Can you work these out from the model? Positions are in its coordinate system, mm. A direction names the side the tool comes from. Round coordinates to 2 decimals unless told otherwise and drop trailing zeros. Loops run counter-clockwise (first coordinate to the right, second up) from the corner with the lowest first, then second, coordinate; pieces in that order, holes last.
Autodesk Inventor part; units mm, degrees
ref_plane "YZ Plane" through (0, 0, 0) normal (1, 0, 0) x (0, 1, 0)
ref_plane "XZ Plane" through (0, 0, 0) normal (0, 1, 0) x (-1, 0, 0)
ref_plane "XY Plane" through (0, 0, 0) normal (0, 0, 1) x (1, 0, 0)
sketch "Sketch1" plane through (0, 0, 0) normal (0, 1, 0) x (-1, 0, 0)
  line L0 (-114.3, 114.3) -> (114.3, 114.3)
  line L1 (114.3, 114.3) -> (114.3, -114.3)
  line L2 (114.3, -114.3) -> (-114.3, -114.3)
  line L3 (-114.3, -114.3) -> (-114.3, 114.3)
  line L4 (-114.3, 114.3) -> (114.3, -114.3) construction
  line L5 (114.3, 114.3) -> (-114.3, -114.3) construction
  line L6 (114.3, 114.3) -> (38.1, 114.3)
  line L7 (38.1, 114.3) -> (38.1, 76.2) construction
  line L8 (38.1, 76.2) -> (114.3, 76.2) construction
  line L9 (114.3, 76.2) -> (114.3, 114.3)
  circle A0 centre (38.1, 76.2) radius 1.5875
  line L10 (114.3, 0) -> (47.3217, 0)
  line L11 (-114.3, 114.3) -> (-38.1, 114.3)
  line L12 (-38.1, 114.3) -> (-38.1, 76.2) construction
  line L13 (-38.1, 76.2) -> (-114.3, 76.2) construction
  line L14 (-114.3, 76.2) -> (-114.3, 114.3)
  circle A1 centre (-38.1, 76.2) radius 1.5875
  line L15 (-114.3, -114.3) -> (-38.1, -114.3)
  line L16 (-38.1, -114.3) -> (-38.1, -76.2) construction
  line L17 (-38.1, -76.2) -> (-114.3, -76.2) construction
  line L18 (-114.3, -76.2) -> (-114.3, -114.3)
  line L19 (114.3, -114.3) -> (38.1, -114.3)
  line L20 (38.1, -114.3) -> (38.1, -76.2) construction
  line L21 (38.1, -76.2) -> (114.3, -76.2) construction
  line L22 (114.3, -76.2) -> (114.3, -114.3)
  circle A2 centre (-38.1, -76.2) radius 1.5875
  circle A3 centre (38.1, -76.2) radius 1.5875
  point P0 (0, 0)
  dimension "d0" = 228.6
  dimension "d1" = 228.6
  dimension "d2" = 76.2
  dimension "d3" = 38.1
  dimension "d4" = 3.175
  dimension "d5" = 76.2
  dimension "d6" = 3.175
  dimension "d7" = 38.1
  dimension "d8" = 76.2
  dimension "d9" = 3.175
  dimension "d10" = 3.175
extrude "Extrusion1" add sketch "Sketch1" along normal blind 12.7
fillet "Fillet1" radius 3.175 4 edges at (-114.3, 6.35, 114.3) (114.3, 6.35, 114.3) (114.3, 6.35, -114.3) (-114.3, 6.35, -114.3)
sketch "Sketch4" plane through (0, 12.7, 0) normal (0, 1, 0) x (1, 0, 0)
  circle A0 centre (-38.1, 76.2) radius 1.5875
  circle A1 centre (38.1, 76.2) radius 1.5875
  circle A2 centre (38.1, -76.2) radius 1.5875
  circle A3 centre (-38.1, -76.2) radius 1.5875
  arc A4 (-111.125, 114.3) -> (-114.3, 111.125) centre (-111.125, 111.125) ccw
  line L0 (-114.3, 111.125) -> (-114.3, -111.125)
  arc A5 (-114.3, -111.125) -> (-111.125, -114.3) centre (-111.125, -111.125) ccw
  line L1 (-111.125, -114.3) -> (111.125, -114.3)
  arc A6 (111.125, -114.3) -> (114.3, -111.125) centre (111.125, -111.125) ccw
  line L2 (114.3, -111.125) -> (114.3, 111.125)
  arc A7 (114.3, 111.125) -> (111.125, 114.3) centre (111.125, 111.125) ccw
  line L3 (111.125, 114.3) -> (-111.125, 114.3)
  line L4 (114.3, 114.3) -> (73.025, 114.3) construction
  line L5 (73.025, 114.3) -> (73.025, 107.95) construction
  line L6 (73.025, 107.95) -> (114.3, 107.95) construction
  line L7 (114.3, 107.95) -> (114.3, 114.3) construction
  line L8 (114.3, 114.3) -> (73.025, 114.3) construction
  line L9 (73.025, 114.3) -> (73.025, 57.15) construction
  line L10 (73.025, 57.15) -> (114.3, 57.15) construction
  line L11 (114.3, 57.15) -> (114.3, 114.3) construction
  circle A8 centre (73.025, 57.15) radius 1.5875
  circle A9 centre (73.025, 107.95) radius 1.5875
  point P0 (0, 0)
  dimension "d22" = 41.275
  dimension "d23" = 6.35
  dimension "d24" = 57.15
  dimension "d25" = 3.175
  dimension "d26" = 3.175
extrude "camMount" cut sketch "Sketch4" against normal up to surface (12.7 mm away) contours A8 | A9
sketch "Sketch5" plane through (0, 12.7, 0) normal (0, 1, 0) x (1, 0, 0)
  circle A0 centre (73.025, 57.15) radius 1.5875 construction
  circle A1 centre (73.025, 107.95) radius 1.5875 construction
  circle A2 centre (-38.1, 76.2) radius 1.5875 construction
  circle A3 centre (38.1, 76.2) radius 1.5875 construction
  circle A4 centre (38.1, -76.2) radius 1.5875 construction
  circle A5 centre (-38.1, -76.2) radius 1.5875 construction
  arc A6 (-111.125, 114.3) -> (-114.3, 111.125) centre (-111.125, 111.125) ccw construction
  line L0 (-114.3, 111.125) -> (-114.3, -111.125) construction
  arc A7 (-114.3, -111.125) -> (-111.125, -114.3) centre (-111.125, -111.125) ccw construction
  line L1 (-111.125, -114.3) -> (111.125, -114.3) construction
  arc A8 (111.125, -114.3) -> (114.3, -111.125) centre (111.125, -111.125) ccw construction
  line L2 (114.3, -111.125) -> (114.3, 111.125) construction
  arc A9 (114.3, 111.125) -> (111.125, 114.3) centre (111.125, 111.125) ccw construction
  line L3 (111.125, 114.3) -> (-111.125, 114.3) construction
  line L4 (114.3, -114.3) -> (107.95, -114.3) construction
  line L5 (107.95, -77.089) -> (114.3, -77.089) construction
  line L6 (114.3, -77.089) -> (114.3, -114.3) construction
  line L7 (114.3, -114.3) -> (59.6392, -114.3) construction
  line L8 (59.6392, -77.089) -> (114.3, -77.089) construction
  line L9 (114.3, -77.089) -> (114.3, -114.3) construction
  line L10 (114.3, -114.3) -> (27.8892, -114.3) construction
  line L11 (27.8892, -114.3) -> (27.8892, -77.089) construction
  line L12 (27.8892, -77.089) -> (114.3, -77.089) construction
  line L13 (114.3, -77.089) -> (114.3, -114.3) construction
  line L14 (114.3, -114.3) -> (76.2, -114.3) construction
  line L15 (76.2, -114.3) -> (76.2, -77.089) construction
  line L16 (76.2, -77.089) -> (114.3, -77.089) construction
  line L17 (114.3, -77.089) -> (114.3, -114.3) construction
  circle A10 centre (76.2, -77.089) radius 1.5875 construction
  circle A11 centre (76.2, -77.089) radius 1.5875
  circle A12 centre (27.8892, -77.089) radius 1.5875
  point P0 (0, 0)
  dimension "d29" = 6.35
  dimension "d30" = 37.211
  dimension "d31" = 54.6608
  dimension "d36" = 86.4108
  dimension "d37" = 38.1
  dimension "d38" = 3.175
extrude "TilitMount" cut sketch "Sketch5" against normal up to surface (12.7 mm away)
sketch "Sketch6" plane through (0, 12.7, 0) normal (0, 1, 0) x (1, 0, 0)
  line L0 (38.1, -95.25) -> (-38.1, -95.25)
  line L1 (-38.1, -95.25) -> (-38.1, 95.25)
  line L2 (-38.1, 95.25) -> (38.1, 95.25)
  line L3 (38.1, 95.25) -> (38.1, -95.25)
  line L4 (38.1, -95.25) -> (-38.1, 95.25) construction
  line L5 (-38.1, -95.25) -> (38.1, 95.25) construction
  line L6 (-38.1, -95.25) -> (38.1, -95.25) construction
  line L7 (-38.1, -101.6) -> (38.1, -101.6)
  line L8 (38.1, -88.9) -> (-38.1, -88.9)
  arc A0 (-38.1, -88.9) -> (-38.1, -101.6) centre (-38.1, -95.25) ccw
  arc A1 (38.1, -101.6) -> (38.1, -88.9) centre (38.1, -95.25) ccw
  line L9 (-38.1, 95.25) -> (38.1, 95.25) construction
  line L10 (-38.1, 88.9) -> (38.1, 88.9)
  line L11 (38.1, 101.6) -> (-38.1, 101.6)
  arc A2 (-38.1, 101.6) -> (-38.1, 88.9) centre (-38.1, 95.25) ccw
  arc A3 (38.1, 88.9) -> (38.1, 101.6) centre (38.1, 95.25) ccw
  line L12 (38.1, -38.1) -> (-38.1, -38.1)
  line L13 (-38.1, -38.1) -> (-38.1, 38.1)
  line L14 (-38.1, 38.1) -> (38.1, 38.1)
  line L15 (38.1, 38.1) -> (38.1, -38.1)
  line L16 (38.1, -38.1) -> (-38.1, 38.1) construction
  line L17 (-38.1, -38.1) -> (38.1, 38.1) construction
  line L18 (38.1, -38.1) -> (38.1, 38.1) construction
  line L19 (44.45, -38.1) -> (44.45, 38.1)
  line L20 (31.75, 38.1) -> (31.75, -38.1)
  arc A4 (31.75, -38.1) -> (44.45, -38.1) centre (38.1, -38.1) ccw
  arc A5 (44.45, 38.1) -> (31.75, 38.1) centre (38.1, 38.1) ccw
  line L21 (-38.1, -38.1) -> (-38.1, 38.1) construction
  line L22 (-31.75, -38.1) -> (-31.75, 38.1)
  line L23 (-44.45, 38.1) -> (-44.45, -38.1)
  arc A6 (-44.45, -38.1) -> (-31.75, -38.1) centre (-38.1, -38.1) ccw
  arc A7 (-31.75, 38.1) -> (-44.45, 38.1) centre (-38.1, 38.1) ccw
  point P0 (0, 0)
  point P1 (0, -95.25)
  point P2 (0, 95.25)
  point P3 (38.1, 0)
  point P4 (-38.1, 0)
  dimension "d39" = 76.2
  dimension "d40" = 190.5
  dimension "d41" = 12.7
  dimension "d42" = 12.7
  dimension "d43" = 76.2
  dimension "d44" = 12.7
  dimension "d45" = 12.7
extrude "Extrusion6" cut sketch "Sketch6" against normal blind 25.4 contours L3 A1 L7 A0 L1 L0 | L0 L1 L8 L3 | A4 L12 L3 | L3 A5 L19 A4 | A6 L23 A7 L1 | L1 L12 A6 | L12 L20 L14 L3 | L1 L14 L22 L12 | L14 A5 L3 | L1 A7 L14 | L10 L1 L2 L3 | L3 L2 L1 A2 L11 A3
sketch "Sketch7" plane through (0, 12.7, 0) normal (0, 1, 0) x (1, 0, 0)
  line L0 (114.3, -111.125) -> (114.3, 111.125)
  line L1 (114.3, 0) -> (104.775, 0)
  line L2 (109.5375, 0) -> (109.5375, 12.7)
  circle A0 centre (109.5375, 12.7) radius 1.5875
  circle A1 centre (109.5375, -12.7) radius 1.5875
  point P0 (0, 0)
  dimension "d48" = 9.525
  dimension "d49" = 12.7
  dimension "d50" = 3.175
extrude "Extrusion7" cut sketch "Sketch7" against normal blind 25.4
sketch "Sketch8" plane through (0, 12.7, 0) normal (0, 1, 0) x (1, 0, 0)
  circle A0 centre (109.5375, -12.7) radius 1.5875
  circle A1 centre (109.5375, -12.7) radius 1.5875 construction
  line L0 (109.5375, -12.7) -> (109.5375, -50.8) construction
  line L1 (109.5375, -50.8) -> (109.5375, -76.2) construction
  circle A2 centre (109.5375, -50.8) radius 1.5875
  circle A3 centre (109.5375, -76.2) radius 1.5875
  line L2 (114.3, 111.125) -> (114.3, -111.125)
  line L3 (114.3, 0) -> (96.6606, 0)
  circle A4 centre (109.5375, 50.8) radius 1.5875
  circle A5 centre (109.5375, 76.2) radius 1.5875
  point P0 (0, 0)
  dimension "d53" = 38.1
  dimension "d54" = 25.4
  dimension "d55" = 3.175
  dimension "d56" = 3.175
extrude "Extrusion8" cut sketch "Sketch8" against normal blind 25.4 contours A2 | A3 | A4 | A5
properties part number "TopPlateV1" material "Polyethylene, High Density"
(1) Suppose I cut it at C-C (y = 7.75). Give the number of separate pieces and of enclosed holes in the cut face, then the cut area to 3 significant figures.
(2) Suppose I cut it at A-A (z = -34). Write out the boundary of the cut face in (x, y), then the cut area to 3 significant figures.
(3) We'd pull the mould along Z, two halves only. Please class faces 1 (the flat face through (-2, 6, -114.3)), 2 (the cylindrical face through (38.24, 6.44, -44.45)), 3 (the flat face through (114.3, 6, -2)), 4 (the cylindrical face through (44.45, 6.44, 95.39)): released by +Z, released by -Z, zero draft, split by the parting line, or undercut.
(4) If I drill on line 1 (X direction, y = 9.5, z = 26); line 2 (Z direction, x = 38.1, y = 4.25); line 3 (Z direction, x = -14.5, y = 5.25), over which ranges is the centre line in solid material (lowest first)?
(5) Suppose I cut it at B-B (z = -95.25). Write out the boundary of the cut face in (x, y), then the cut area to 3 significant figures.
(6) Which directions (+Z, -Z, +X, -X, +Y, -Y) give clear straight access to the entire face, cutting with the end or side of a thin tool? Please do faces 5 (the flat face through (2, 6, 114.3)), 6 (the flat face through (-1, 6, -88.9)).
Check result:
1. separate pieces: 1
1. enclosed holes: 18
1. area: 47,800 mm2
2. outline: (-114.3, 0) - (-44.45, 0) - (-44.45, 12.7) - (-114.3, 12.7) - close; (-31.75, 0) - (31.75, 0) - (31.75, 12.7) - (-31.75, 12.7) - close; (44.45, 0) - (114.3, 0) - (114.3, 12.7) - (44.45, 12.7) - close
2. area: 2,580 mm2
3. face 1: released by -Z
3. face 2: undercut
3. face 3: zero draft
3. face 4: undercut
4. line 1: x = -114.3 to -44.45, -31.75 to 31.75, 44.45 to 114.3
4. line 2: z = -114.3 to -101.6, -88.9 to -77.79, -74.61 to -44.45, 44.45 to 74.61, 77.79 to 88.9, 101.6 to 114.3
4. line 3: z = -114.3 to -101.6, -88.9 to 88.9, 101.6 to 114.3
5. outline: (-114.3, 0) - (-44.45, 0) - (-44.45, 12.7) - (-114.3, 12.7) - close; (44.45, 0) - (114.3, 0) - (114.3, 12.7) - (44.45, 12.7) - close
5. area: 1,770 mm2
6. face 5: +Z, +X, -X, +Y, -Y
6. face 6: +Y, -Y
